Model file for the job. Use its own axes, mm. Face numbers are marked on the shaded views. A direction names the side the tool comes from. Give positions to 0.01 mm unless a question says otherwise; leave off trailing zeros. Loops run counter-clockwise (first coordinate to the right, second up) from the corner with the lowest first, then second, coordinate; pieces in that order, holes last. Notation, with made-up numbers: M 19,-7 L 33,-7 A13 cw 33,12 Z; hole C -25,-8.75 d4. An arc over 180 degrees is marked long. Answer in a Markdown table with one row per item.
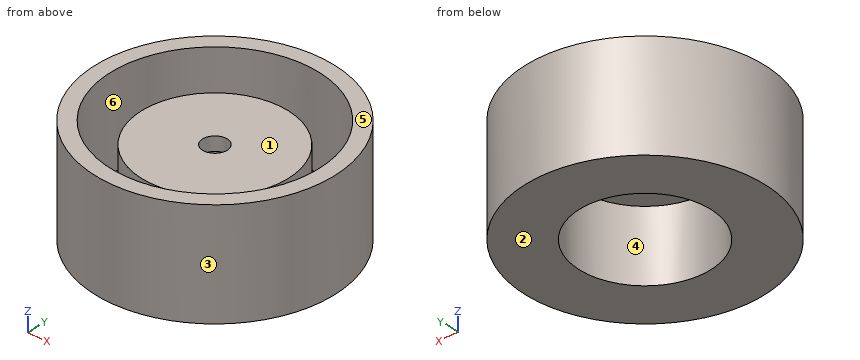
```python
from build123d import *

# Parameters (mm, degrees)
SKETCH1_R           = 19.685
BOSS_EXTRUDE4_DEPTH = 17.526
SHELL1_T            = -2.54
SKETCH2_R           = 12.065
BOSS_EXTRUDE5_DEPTH = 11.43
SKETCH3_R           = 10.795
CUT_EXTRUDE1_DEPTH  = 11.684
SKETCH4_R           = 2.032
CUT_EXTRUDE2_DEPTH  = 2.54


with BuildPart() as part:
    # Sketch1 → Boss-Extrude4 (new body)
    with BuildSketch(Plane.XY):
        with Locations((-69.769461907, 37.477045181)):
            Circle(SKETCH1_R)
    extrude(amount=BOSS_EXTRUDE4_DEPTH)

    # Shell1
    shell1_openings = [part.faces().sort_by_distance(p)[0] for p in [
        (-69.769461907, 37.477045181, 17.526),
    ]]
    offset(amount=SHELL1_T, openings=shell1_openings, kind=Kind.INTERSECTION)

    # Sketch2 → Boss-Extrude5 (add)
    with BuildSketch(Plane.XY.offset(2.54)):
        with Locations((-69.769461907, 37.477045181)):
            Circle(SKETCH2_R)
    extrude(amount=BOSS_EXTRUDE5_DEPTH)

    # Sketch3 → Cut-Extrude1 (cut)
    with BuildSketch(Plane(origin=(0, 0, 0), x_dir=(-1, 0, 0), z_dir=(0, 0, -1))):
        with Locations((69.769461907, 37.477045181)):
            Circle(SKETCH3_R)
    extrude(amount=-CUT_EXTRUDE1_DEPTH, mode=Mode.SUBTRACT)

    # Sketch4 → Cut-Extrude2 (cut)
    with BuildSketch(Plane.XY.offset(13.97)):
        with Locations((-69.769461907, 37.477045181)):
            Circle(SKETCH4_R)
    extrude(amount=-CUT_EXTRUDE2_DEPTH, mode=Mode.SUBTRACT)


solid = part.part
```
(1) Wall check: L1, parallel to X at y = 32, z = 4.5; L2, parallel to Y at x = -63, z = 6; L3, parallel to Y at x = -73, z = 3.5. Give the ranges that are in metal, low to high.
Established:
| item | result |
|---|---|
| L1 | x = -88.68 to -86.02, -80.52 to -79.07, -60.47 to -59.02, -53.52 to -50.86 |
| L2 | y = 18.99 to 21.73, 27.49 to 29.07, 45.89 to 47.46, 53.23 to 55.96 |
| L3 | y = 18.06 to 20.64, 25.85 to 27.18, 47.78 to 49.1, 54.31 to 56.9 |
(2) Which spindle directions (+Z, -Z, +X, -X, +Y, -Y) get a long thin tool onto all of the face, cutting with end or side? Do the marked faces 1 and 2. Say none if no direction does.
Established:
| item | result |
|---|---|
| face 1 | +Z |
| face 2 | -Z, +X, -X, +Y, -Y |
(3) Saw through at B-B, the plane z = 5.25. Give the cut face in (x, y) (3 decimals).
Established:
| item | result |
|---|---|
| outline | C -69.769,37.477 d39.37; C -69.769,37.477 d24.13; hole C -69.769,37.477 d34.29; hole C -69.769,37.477 d21.59 |
(4) Flat gauge pins, fed straight in: P1, Ø11, axis at x = -74.5, y = 38, coming from the -Z side; P2, Ø3.5, axis at x = -69.77, y = 37.48, coming from the +Z side; P3, Ø10.5, axis at x = -66, y = 44.5, coming from the +Z side; P4, Ø4, axis at x = -55, y = 36, coming from the +Z side. Where does each tip first touch, or does it go through?
Established:
| item | result |
|---|---|
| P1 | stops at z = 11.68 |
| P2 | passes through |
| P3 | stops at z = 13.97 |
| P4 | stops at z = 2.54 |
(5) Saw through at D-D, the plane y = 32. Give the cut face in (x, z).
Established:
| item | result |
|---|---|
| outline | M -88.68,0 L -79.07,0 L -79.07,11.68 L -60.47,11.68 L -60.47,0 L -50.86,0 L -50.86,17.53 L -53.52,17.53 L -53.52,2.54 L -59.02,2.54 L -59.02,13.97 L -80.52,13.97 L -80.52,2.54 L -86.02,2.54 L -86.02,17.53 L -88.68,17.53 Z |
(6) Saw through at C-C, the plane x = -64. Give the cut face in (y, z).
Established:
| item | result |
|---|---|
| outline | M 18.66,0 L 28.35,0 L 28.35,11.68 L 46.6,11.68 L 46.6,0 L 56.3,0 L 56.3,17.53 L 53.62,17.53 L 53.62,2.54 L 48.07,2.54 L 48.07,13.97 L 26.88,13.97 L 26.88,2.54 L 21.33,2.54 L 21.33,17.53 L 18.66,17.53 Z |
(7) Saw through at A-A, the plane y = 37. Give the cut face in (x, z) (3 decimals), and give its area (3 significant figures).
Established:
| item | result |
|---|---|
| outline | M -89.449,0 L -80.554,0 L -80.554,11.684 L -71.745,11.684 L -71.745,13.97 L -81.825,13.97 L -81.825,2.54 L -86.908,2.54 L -86.908,17.526 L -89.449,17.526 Z; M -67.794,11.684 L -58.985,11.684 L -58.985,0 L -50.09,0 L -50.09,17.526 L -52.631,17.526 L -52.631,2.54 L -57.714,2.54 L -57.714,13.97 L -67.794,13.97 Z |
| area | 191 mm2 |
(8) Mould opens along Y. For the marked faces 3, 4, 5 and 6 say: pulls with the +Y half, pulls with the -Y half, needs draft (parallel to the pull), parting line crosses it, or undercut.
Established:
| item | result |
|---|---|
| face 3 | parting line crosses it |
| face 4 | undercut |
| face 5 | needs draft |
| face 6 | undercut |
